Model file for the job. Use its own axes, mm. A direction names the side the tool comes from. Round coordinates to 2 decimals unless told otherwise and drop trailing zeros. Order: outer loops, then holes, each group sorted by start corner. A loop starts at its lowest first (then second) coordinate and runs counter-clockwise, first axis right, second up. Notation, with made-up numbers: (-21, 56) - (35, 56) arc R9 cw to (35, 62) - close; hole circle Ø5 at (-22.5, -28.5). An arc over 180 degrees is marked (long way). Write item = value, one per line.
```python
from build123d import *

# Parameters (mm, degrees)
SM_BASE_FLANGE_1_DEPTH = 394
SKETCH_6_W             = 40
SKETCH_6_H             = 80
CUT_EXTRUDE_1_DEPTH    = 4
SKETCH_8_W             = 13
SKETCH_8_H             = 60
CUT_EXTRUDE_2_DEPTH    = 24
SKETCH_9_W             = 35
SKETCH_9_H             = 33
CUT_EXTRUDE_3_DEPTH    = 4
SKETCH_10_R            = 8.25
SKETCH_10_R_2          = 3.25
SKETCH_10_R_3          = 2.5
CUT_EXTRUDE_4_DEPTH    = 10
SKETCH_11_R            = 2.5
SKETCH_11_R_2          = 3.25
CUT_EXTRUDE_5_DEPTH    = 10
CUT_EXTRUDE_6_DEPTH    = 10
OTHER_START            = 229.809703886
OTHER_1_OUTLINE_W      = 445.809703886
OTHER_1_OUTLINE_H      = 4
OTHER_1_DEPTH          = 3.535533906
OTHER_START_2          = -214.2533547
OTHER_1_2_OUTLINE_W    = 4.190296114
OTHER_1_2_OUTLINE_H    = 4
OTHER_1_2_DEPTH        = 7.071067812


# Read off the part's stored shape, not the designer's step: Затупленный угол1
# Sheet-metal steps are written as plain solids
with BuildPart() as part:
    # Sketch 1 → Sm Base Flange 1 (new, symmetric)
    with BuildSketch(Plane.XY):
        with BuildLine():
            Line((0, 0), (-31, 0))
            ThreePointArc((-31, 0), (-33.828427125, 1.171572875), (-35, 4))
            Line((-35, 4), (-35, 96))
            ThreePointArc((-35, 96), (-33.828427125, 98.828427125), (-31, 100))
            Line((-31, 100), (-26, 100))
            ThreePointArc((-26, 100), (-24.585786438, 100.585786438), (-24, 102))
            Line((-24, 102), (-24, 120))
            ThreePointArc((-24, 120), (-22.828427125, 122.828427125), (-20, 124))
            Line((-20, 124), (16, 124))
            Line((16, 124), (16, 122))
            Line((16, 122), (-20, 122))
            ThreePointArc((-20, 122), (-21.414213562, 121.414213562), (-22, 120))
            Line((-22, 120), (-22, 102))
            ThreePointArc((-22, 102), (-23.171572875, 99.171572875), (-26, 98))
            Line((-26, 98), (-31, 98))
            ThreePointArc((-31, 98), (-32.414213562, 97.414213562), (-33, 96))
            Line((-33, 96), (-33, 4))
            ThreePointArc((-33, 4), (-32.414213562, 2.585786438), (-31, 2))
            Line((-31, 2), (0, 2))
            Line((0, 2), (0, 0))
        make_face()
    extrude(amount=SM_BASE_FLANGE_1_DEPTH, both=True)

    # Эскиз6 → Вырез-Вытянуть1 (cut)
    with BuildSketch(Plane(origin=(0, 124, 0), x_dir=(1, 0, 0), z_dir=(0, 1, 0))):
        with Locations((-4, -354)):
            Rectangle(SKETCH_6_W, SKETCH_6_H)
        with Locations((-4, 354)):
            Rectangle(SKETCH_6_W, SKETCH_6_H)
    extrude(amount=-CUT_EXTRUDE_1_DEPTH, mode=Mode.SUBTRACT)

    # Эскиз8 → Вырез-Вытянуть2 (cut)
    with BuildSketch(Plane(origin=(0, 120, 0), x_dir=(1, 0, 0), z_dir=(0, 1, 0))):
        with Locations((-28.5, 364)):
            Rectangle(SKETCH_8_W, SKETCH_8_H)
        with Locations((-28.5, -364)):
            Rectangle(SKETCH_8_W, SKETCH_8_H)
    extrude(amount=-CUT_EXTRUDE_2_DEPTH, mode=Mode.SUBTRACT)

    # Эскиз9 → Вырез-Вытянуть3 (cut)
    with BuildSketch(Plane.XZ):
        with Locations((-17.5, -377.5)):
            Rectangle(SKETCH_9_W, SKETCH_9_H)
        with Locations((-17.5, 377.5)):
            Rectangle(SKETCH_9_W, SKETCH_9_H)
    extrude(amount=-CUT_EXTRUDE_3_DEPTH, mode=Mode.SUBTRACT)

    # Эскиз10 → Вырез-Вытянуть4 (cut)
    with BuildSketch(Plane.ZY.offset(35)):
        with Locations((-365, 50)):
            Circle(SKETCH_10_R)
        with Locations((-365, 20)):
            Circle(SKETCH_10_R_2)
        with Locations((-365, 70)):
            Circle(SKETCH_10_R_2)
        with Locations((-285, 20)):
            Circle(SKETCH_10_R_2)
        with Locations((-285, 70)):
            Circle(SKETCH_10_R_2)
        with Locations((-325, 50)):
            Circle(SKETCH_10_R)
        with Locations(Location((325, 50, 0), (0, 0, 180))):
            Circle(SKETCH_10_R)
        with Locations(Location((285, 70, 0), (0, 0, 180))):
            Circle(SKETCH_10_R_2)
        with Locations(Location((285, 20, 0), (0, 0, 180))):
            Circle(SKETCH_10_R_2)
        with Locations(Location((365, 70, 0), (0, 0, 180))):
            Circle(SKETCH_10_R_2)
        with Locations(Location((365, 20, 0), (0, 0, 180))):
            Circle(SKETCH_10_R_2)
        with Locations(Location((365, 50, 0), (0, 0, 180))):
            Circle(SKETCH_10_R)
        with Locations((-250, 50)):
            Circle(SKETCH_10_R_3)
        with Locations((0, 50)):
            Circle(SKETCH_10_R_3)
        with Locations((250, 50)):
            Circle(SKETCH_10_R_3)
    extrude(amount=-CUT_EXTRUDE_4_DEPTH, mode=Mode.SUBTRACT)

    # Эскиз11 → Вырез-Вытянуть5 (cut)
    with BuildSketch(Plane.ZY.offset(24)):
        with Locations((300, 110)):
            Circle(SKETCH_11_R)
        with Locations((275, 110)):
            Circle(SKETCH_11_R)
        with Locations((250, 110)):
            Circle(SKETCH_11_R)
        with Locations((225, 110)):
            Circle(SKETCH_11_R)
        with Locations((322, 113)):
            Circle(SKETCH_11_R_2)
        with Locations(Location((-322, 113, 0), (0, 0, 180))):
            Circle(SKETCH_11_R_2)
        with Locations(Location((-225, 110, 0), (0, 0, 180))):
            Circle(SKETCH_11_R)
        with Locations(Location((-250, 110, 0), (0, 0, 180))):
            Circle(SKETCH_11_R)
        with Locations(Location((-275, 110, 0), (0, 0, 180))):
            Circle(SKETCH_11_R)
        with Locations(Location((-300, 110, 0), (0, 0, 180))):
            Circle(SKETCH_11_R)
    extrude(amount=-CUT_EXTRUDE_5_DEPTH, mode=Mode.SUBTRACT)

    # Эскиз12 → Вырез-Вытянуть6 (cut)
    with BuildSketch(Plane(origin=(0, 124, 0), x_dir=(1, 0, 0), z_dir=(0, 1, 0))):
        with BuildLine():
            Line((-4.5, 235.5), (-4.5, 264.5))
            ThreePointArc((-4.5, 264.5), (1, 270), (6.5, 264.5))
            Line((6.5, 264.5), (6.5, 235.5))
            ThreePointArc((6.5, 235.5), (1, 230), (-4.5, 235.5))
        make_face()
        with BuildLine():
            Line((-4.5, -14.5), (-4.5, 14.5))
            ThreePointArc((-4.5, 14.5), (1, 20), (6.5, 14.5))
            Line((6.5, 14.5), (6.5, -14.5))
            ThreePointArc((6.5, -14.5), (1, -20), (-4.5, -14.5))
        make_face()
        with BuildLine():
            Line((-4.5, 35.5), (-4.5, 64.5))
            ThreePointArc((-4.5, 64.5), (1, 70), (6.5, 64.5))
            Line((6.5, 64.5), (6.5, 35.5))
            ThreePointArc((6.5, 35.5), (1, 30), (-4.5, 35.5))
        make_face()
        with BuildLine():
            Line((-4.5, 85.5), (-4.5, 114.5))
            ThreePointArc((-4.5, 114.5), (1, 120), (6.5, 114.5))
            Line((6.5, 114.5), (6.5, 85.5))
            ThreePointArc((6.5, 85.5), (1, 80), (-4.5, 85.5))
        make_face()
        with BuildLine():
            Line((-4.5, 135.5), (-4.5, 164.5))
            ThreePointArc((-4.5, 164.5), (1, 170), (6.5, 164.5))
            Line((6.5, 164.5), (6.5, 135.5))
            ThreePointArc((6.5, 135.5), (1, 130), (-4.5, 135.5))
        make_face()
        with BuildLine():
            Line((-4.5, 185.5), (-4.5, 214.5))
            ThreePointArc((-4.5, 214.5), (1, 220), (6.5, 214.5))
            Line((6.5, 214.5), (6.5, 185.5))
            ThreePointArc((6.5, 185.5), (1, 180), (-4.5, 185.5))
        make_face()
        with BuildLine():
            Line((-4.5, -64.5), (-4.5, -35.5))
            ThreePointArc((-4.5, -35.5), (1, -30), (6.5, -35.5))
            Line((6.5, -35.5), (6.5, -64.5))
            ThreePointArc((6.5, -64.5), (1, -70), (-4.5, -64.5))
        make_face()
        with BuildLine():
            Line((-4.5, -114.5), (-4.5, -85.5))
            ThreePointArc((-4.5, -85.5), (1, -80), (6.5, -85.5))
            Line((6.5, -85.5), (6.5, -114.5))
            ThreePointArc((6.5, -114.5), (1, -120), (-4.5, -114.5))
        make_face()
        with BuildLine():
            Line((-4.5, -164.5), (-4.5, -135.5))
            ThreePointArc((-4.5, -135.5), (1, -130), (6.5, -135.5))
            Line((6.5, -135.5), (6.5, -164.5))
            ThreePointArc((6.5, -164.5), (1, -170), (-4.5, -164.5))
        make_face()
        with BuildLine():
            Line((-4.5, -214.5), (-4.5, -185.5))
            ThreePointArc((-4.5, -185.5), (1, -180), (6.5, -185.5))
            Line((6.5, -185.5), (6.5, -214.5))
            ThreePointArc((6.5, -214.5), (1, -220), (-4.5, -214.5))
        make_face()
        with BuildLine():
            Line((-4.5, -264.5), (-4.5, -235.5))
            ThreePointArc((-4.5, -235.5), (1, -230), (6.5, -235.5))
            Line((6.5, -235.5), (6.5, -264.5))
            ThreePointArc((6.5, -264.5), (1, -270), (-4.5, -264.5))
        make_face()
    extrude(amount=-CUT_EXTRUDE_6_DEPTH, mode=Mode.SUBTRACT)

    # Other 1 outline → Other 1 (cut)
    with BuildSketch(Plane(origin=(0, 0, 0), x_dir=(0.707106781186546, 0, -0.707106781186549), z_dir=(0.707106781186549, 0, 0.707106781186546)).offset(OTHER_START)):
        with Locations((6.904851943, 123)):
            Rectangle(OTHER_1_OUTLINE_W, OTHER_1_OUTLINE_H)
    extrude(amount=OTHER_1_DEPTH, mode=Mode.SUBTRACT)

    # Other 1 2 outline → Other 1 2 (cut)
    with BuildSketch(Plane(origin=(0, 0, 0), x_dir=(0.707106781186546, 0, -0.707106781186549), z_dir=(0.707106781186549, 0, 0.707106781186546)).offset(OTHER_START_2)):
        with Locations((231.904851943, 123)):
            Rectangle(OTHER_1_2_OUTLINE_W, OTHER_1_2_OUTLINE_H)
    extrude(amount=OTHER_1_2_DEPTH, mode=Mode.SUBTRACT)


solid = part.part
```
1) Cut at B-B (x = -12). Write the cut outline in (y, z), and give its area (3 significant figures).
Conclusion:
outline = (0, -361) - (2, -361) - (2, 361) - (0, 361) - close; (122, -314) - (124, -314) - (124, 314) - (122, 314) - close
area = 2,700 mm^2
2) 3-axis set-ups, long thin cutter, end or side, ignore diameter. For faces 1 (the face through (-6, 124, 4)), 2 (the face through (-24, 111, 5)), 3 (the face through (-22, 111, 5)): which of +Z, -Z, +X, -X, +Y, -Y reach the whole face in a straight line?
Conclusion:
face_1 = +Z, -Z, +X, -X, +Y
face_2 = +Z, -Z, -X, +Y
face_3 = +Z, -Z, +X
3) Cut at A-A (z = -105). Write the cut outline in (x, y).
Conclusion:
outline = (-35, 4) arc R4 ccw to (-31, 0) - (0, 0) - (0, 2) - (-31, 2) arc R2 cw to (-33, 4) - (-33, 96) arc R2 cw to (-31, 98) - (-26, 98) arc R4 ccw to (-22, 102) - (-22, 120) arc R2 cw to (-20, 122) - (-4.5, 122) - (-4.5, 124) - (-20, 124) arc R4 ccw to (-24, 120) - (-24, 102) arc R2 cw to (-26, 100) - (-31, 100) arc R4 ccw to (-35, 96) - close; (6.5, 122) - (16, 122) - (16, 124) - (6.5, 124) - close
4) Wall check: line 1 along Y through (x, z) = (-17.5, -2); line 2 along Y through (x, z) = (-27.5, -277.5); line 3 along X through (y, z) = (50, -143). Give the ranges that are in metal, low to high.
Conclusion:
line_1 = 0 to 2, 122 to 124
line_2 = 0 to 2, 98 to 100
line_3 = -35 to -33
5) Flat gauge pins, fed straight in: pin 1 Ø10 at (y, z) = (50, -325) entering from +X; pin 2 Ø4.5 at (x, y) = (-21.5, 2) entering from +Z; pin 3 Ø5.5 at (y, z) = (107, -64.5) entering from -X; pin 4 Ø1 at (y, z) = (123, 243.5) entering from -X. Where does each tip first touch, or does it go through?
Conclusion:
pin_1 = through
pin_2 = 361
pin_3 = -24
pin_4 = -23.12
6) Mould opens along Z. For faces 4 (the face through (-6, 122, 4)), 5 (the face through (-23.7, 105.4, 334)), 6 (the face through (-23.7, 105.4, -334)), 7 (the face through (-34.014, 49.637, 373.242)) say: +Z half, -Z half, draft (parallel to the pull), parting line (faces both ways), or undercut.
Conclusion:
face_4 = draft
face_5 = +Z half
face_6 = -Z half
face_7 = undercut
